```python
from build123d import *

# Parameters (mm, degrees)
PAD_DEPTH    = 12
SKETCH002_R  = 2
POCKET_DEPTH = 36.001


with BuildPart() as part:
    # Sketch001 → Pad (new body)
    with BuildSketch(Plane.XY):
        with BuildLine():
            ThreePointArc((0, -6.35), (6.22047, 1.276029), (-2.5, 5.837165))
            ThreePointArc((-4.330691, 10.111633), (-5.552574, 7.059055), (-2.5, 5.837165))
            ThreePointArc((7.698987, -7.856564), (9.14059, 6.11961), (-4.330691, 10.111633))
            Line((7.698987, -7.856564), (-20, -35))
            Line((-25, -35), (-20, -35))
            Line((-25, 20), (-25, -35))
            Line((-20, 20), (-25, 20))
            Line((-20, 0), (-20, 20))
            Line((0, -6.35), (-20, 0))
        make_face()
        Polygon((-20, -5.245966), (-20, -27.999484), (-2.462803, -10.814026), align=None, mode=Mode.SUBTRACT)
    extrude(amount=PAD_DEPTH)

    # Sketch002 → Pocket (cut, through all)
    with BuildSketch(Plane(origin=(-25, 0, 0), x_dir=(0, -1, 0), z_dir=(-1, 0, 0))):
        with Locations((-12, 6)):
            Circle(SKETCH002_R)
        with Locations((16, 6)):
            Circle(SKETCH002_R)
    extrude(amount=-POCKET_DEPTH, mode=Mode.SUBTRACT)


solid = part.part
```
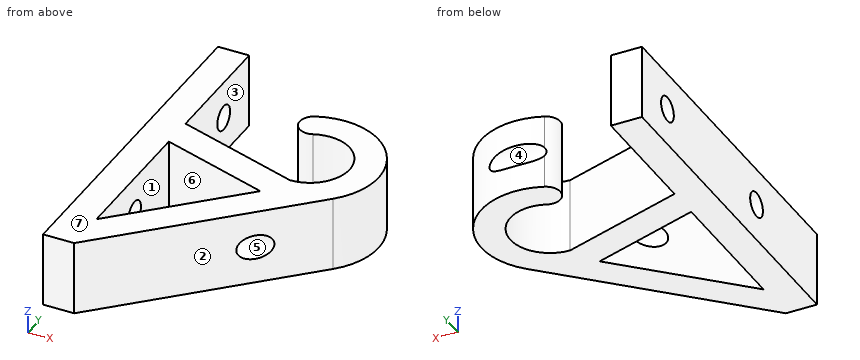
Geometry: final body of the model. Coordinates: model frame, mm. Face numbers are marked on the shaded views. A direction names the side the tool comes from. Coordinates: 2 decimals unless noted, no trailing zeros. Loops run counter-clockwise (first coordinate to the right, second up) from the corner with the lowest first, then second, coordinate; pieces in that order, holes last. Notation, with made-up numbers: (-4, -31.75) -> (43, -31.75) arc R8 cw to (43, -23.75) -> close; hole circle Ø3 at (81, -37.5). An arc over 180 degrees is marked (long way). Use a Markdown table: item, result. Add a question column.
(1) Mould query, pull axis Z, two halves, no side actions, for the marked faces 4, 5, 6 and 7. Classes: pulls with the +Z half, pulls with the -Z half, needs draft (parallel to the pull), parting line crosses it, or undercut.
(2) Section query C-C, the plane y = -16. Return loops of the section in (x, z), plus the area to 3 significant figures.
(3) Pin query (flat end, axial travel): pin 1 Ø6 at (x, z) = (-12, 6) entering from -Y; pin 2 Ø5 at (y, z) = (-28, 6.5) entering from +X; pin 3 Ø6.5 at (y, z) = (-16, 6) entering from +X. Return the tip coordinate at first contact, or that it passes through.
(4) Section query D-D, the plane z = 6. Return loops of the section in (x, y) (3 decimals).
(5) Section query A-A, the plane y = 12. Return loops of the section in (x, z), plus the area to 3 significant figures.
(6) Line query: line 1 along Z through (x, y) = (-23.2, -16); line 2 along Y through (x, z) = (-4, 6.25); line 3 along Y through (x, z) = (-12, 8.25). Output: solid intervals per line, ascending.
(7) Access query for the marked faces 1, 2 and 3. Directions: +Z, -Z, +X, -X, +Y, -Y. A direction counts if a zero-diameter tool reaches every point of the face in a straight line with its end or side. Return the directions, or none.
(8) Section query B-B, the plane x = -10.5. Return loops of the section in (y, z).
Answer:
| question | item | result |
|---|---|---|
| 1 | face 4 | undercut |
| 1 | face 5 | undercut |
| 1 | face 6 | needs draft |
| 1 | face 7 | pulls with the +Z half |
| 2 | outline | (-25, 0) -> (-20, 0) -> (-20, 4) -> (-25, 4) -> close; (-25, 8) -> (-20, 8) -> (-20, 12) -> (-25, 12) -> close; (-7.75, 0) -> (-0.61, 0) -> (-0.61, 4) -> (-7.75, 4) -> close; (-7.75, 8) -> (-0.61, 8) -> (-0.61, 12) -> (-7.75, 12) -> close |
| 2 | area | 97.2 mm^2 |
| 3 | pin 1 | stops at y = -30.1 |
| 3 | pin 2 | stops at x = -10.31 |
| 3 | pin 3 | stops at x = 2.71 |
| 4 | outline | (-25, -35) -> (-20, -35) -> (-2.652, -18) -> (-9.796, -18) -> (-20, -27.999) -> (-20, -18) -> (-25, -18) -> close; (-25, -14) -> (-20, -14) -> (-20, -5.246) -> (-2.463, -10.814) -> (-5.714, -14) -> (1.43, -14) -> (7.699, -7.857) arc R11 ccw to (4.583, 10) -> (-4.557, 10) arc R2.325 ccw to (-2.5, 5.837) arc R6.35 cw (long way) to (0, -6.35) -> (-20, 0) -> (-20, 10) -> (-25, 10) -> close; (-25, 14) -> (-20, 14) -> (-20, 20) -> (-25, 20) -> close |
| 5 | outline | (-25, 0) -> (-20, 0) -> (-20, 4) -> (-25, 4) -> close; (-25, 8) -> (-20, 8) -> (-20, 12) -> (-25, 12) -> close |
| 5 | area | 40.0 mm^2 |
| 6 | line 1 | z = 0 to 4, 8 to 12 |
| 6 | line 2 | y = -19.32 to -17.98, -14.02 to -12.32, -10.33 to -5.08, 5.72 to 10.02 |
| 6 | line 3 | y = -27.16 to -20.16, -7.79 to -2.54 |
| 7 | face 1 | +Z, -Z |
| 7 | face 2 | +Z, -Z, +X, -Y |
| 7 | face 3 | +Z, -Z, +Y |
| 8 | outline | (-25.69, 0) -> (-18.69, 0) -> (-18.69, 12) -> (-25.69, 12) -> close; (-8.26, 0) -> (-3.02, 0) -> (-3.02, 12) -> (-8.26, 12) -> close |
